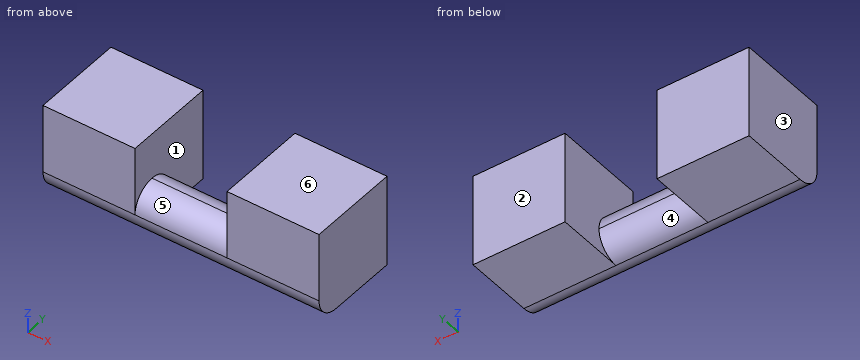
```python
from build123d import *

# Parameters (mm, degrees)
F0_W     = 20
F0_H     = 20
F1_DEPTH = 30
F2_W     = 20
F2_H     = 10
F3_DEPTH = 20
F4_W     = 20
F4_H     = 10
F5_DEPTH = 25
F6_R     = 4.99999


# Not quite as in the source:
# - a fillet or chamfer is up to 0.001 mm smaller than in the source, because OpenCascade refuses the exact size


with BuildPart() as f1:
    # F0 (on Right) → F1 (new body, symmetric)
    with BuildSketch(Plane.YZ):
        Rectangle(F0_W, F0_H)
    extrude(amount=F1_DEPTH, both=True)

    # F2 (on face) → F3 (cut)
    with BuildSketch(Plane.XZ.offset(10)):
        with Locations((0, 5)):
            Rectangle(F2_W, F2_H)
    extrude(amount=-F3_DEPTH, mode=Mode.SUBTRACT)

    # F4 (on face) → F5 (cut)
    with BuildSketch(Plane.XY):
        with Locations((0, 5)):
            Rectangle(F4_W, F4_H)
    extrude(amount=-F5_DEPTH, mode=Mode.SUBTRACT)

    # F6 (radius 5 in the source; OpenCascade refuses exactly that, so slightly less here)
    f6_edges = [f1.edges().sort_by_distance(p)[0] for p in [
        (0, 0, 0),
        (0, 0, -10),
        (0, -10, 0),
        (0, -10, -10),
    ]]
    fillet(f6_edges, radius=F6_R)


solid = f1.part
```
Model file for the job. Use its own axes, mm. Face numbers are marked on the shaded views. A direction names the side the tool comes from. Coordinates: 2 decimals unless noted, no trailing zeros. Loops run counter-clockwise (first coordinate to the right, second up) from the corner with the lowest first, then second, coordinate; pieces in that order, holes last. Notation, with made-up numbers: (-32.75, -39) - (25.25, -39) arc R34 cw to (25.25, 0) - close; hole circle Ø8 at (44.5, 48). An arc over 180 degrees is marked (long way). Write item = value, one per line. Start each with the question number.
Item 1: Drop flat-ended pins along their axis: pin 1 Ø3 at (x, y) = (3.5, -7.5) entering from -Z; pin 2 Ø2 at (x, z) = (-2.5, -7.5) entering from -Y; pin 3 Ø2 at (x, z) = (-4.5, -2.5) entering from +Y. Give the stop position or say it passes through.
Item 2: 3-axis set-ups, long thin cutter, end or side, ignore diameter. For the marked faces 4, 5 and 6: which of +Z, -Z, +X, -X, +Y, -Y reach the whole face in a straight line?
Item 3: Saw through at C-C, the plane z = -6. List the corners of the cut face in (x, y), then the cut area to 3 significant figures.
Item 4: Saw through at D-D, the plane y = -6.5. List the corners of the cut face in (x, z), then the cut area to 3 significant figures.
Item 5: Saw through at A-A, the plane y = 0.75. List the corners of the cut face in (x, z).
Item 6: Pull direction X, two halves, no side cores. Call the marked faces 1, 2 and 3: +X half, -X half, draft (parallel to the pull), parting line (faces both ways), or undercut.
Item 7: Wall check: probe 1 along X at (y, z) = (4.75, -8.5); probe 2 along Y at (x, z) = (-16, -7.25); probe 3 along Y at (x, z) = (12.5, -6.5). Give the ranges that are in metal, low to high. Write a range as [from, to].
Answers:
q1.pin_1 = -9.9
q1.pin_2 = -9.77
q1.pin_3 = -0.23
q2.face_4 = -Z, +Y
q2.face_5 = +Z, -Y
q2.face_6 = +Z, +X, -X, +Y, -Y
q3.outline = (-30, -9.9) - (30, -9.9) - (30, 10) - (10, 10) - (10, -0.1) - (-10, -0.1) - (-10, 10) - (-30, 10) - close
q3.area = 992 mm2
q4.outline = (-30, -9.77) - (30, -9.77) - (30, 10) - (10, 10) - (10, -0.23) - (-10, -0.23) - (-10, 10) - (-30, 10) - close
q4.area = 982 mm2
q5.outline = (-30, -10) - (-10, -10) - (-10, 10) - (-30, 10) - close; (10, -10) - (30, -10) - (30, 10) - (10, 10) - close
q6.face_1 = undercut
q6.face_2 = draft
q6.face_3 = -X half
q7.probe_1 = [-30, -10], [10, 30]
q7.probe_2 = [-9.47, 10]
q7.probe_3 = [-9.77, 10]
